Here's the drawing with two shaded views (mm, measured from the low corner). I have some questions. Round coordinates to 2 decimals unless told otherwise and drop trailing zeros. Loops run counter-clockwise (first coordinate to the right, second up) from the corner with the lowest first, then second, coordinate; pieces in that order, holes last. Notation, with made-up numbers: M -9,-32 L 49,-32 A23 cw 49,-5 Z; hole C 46,-39 d10. An arc over 180 degrees is marked long. One line per item, written item: value. Start each with the question number.
Q1. Please list where these lines run through material, in increasing order: line 1 along Y through (x, z) = (10, 31.5); line 2 along Y through (x, z) = (35, 10.5); line 3 along X through (y, z) = (11, 3.5).
Q2. Imagine slicing it at C-C (z = 8.5). Please give me the cut outline in (x, y), then the cut area to 3 significant figures.
Q3. Imagine slicing it at A-A (x = 10). Please give me the cut outline in (y, z), then the cut area to 3 significant figures.
Q4. Thinking about a two-plate mould opening in Y: for the marked faces 1, 2 and 3, which applies, released by +Y, released by -Y, zero draft, split by the parting line, or undercut?
Q5. Imagine slicing it at B-B (y = 93). Please give me the cut outline in (x, z), then the cut area to 3 significant figures.
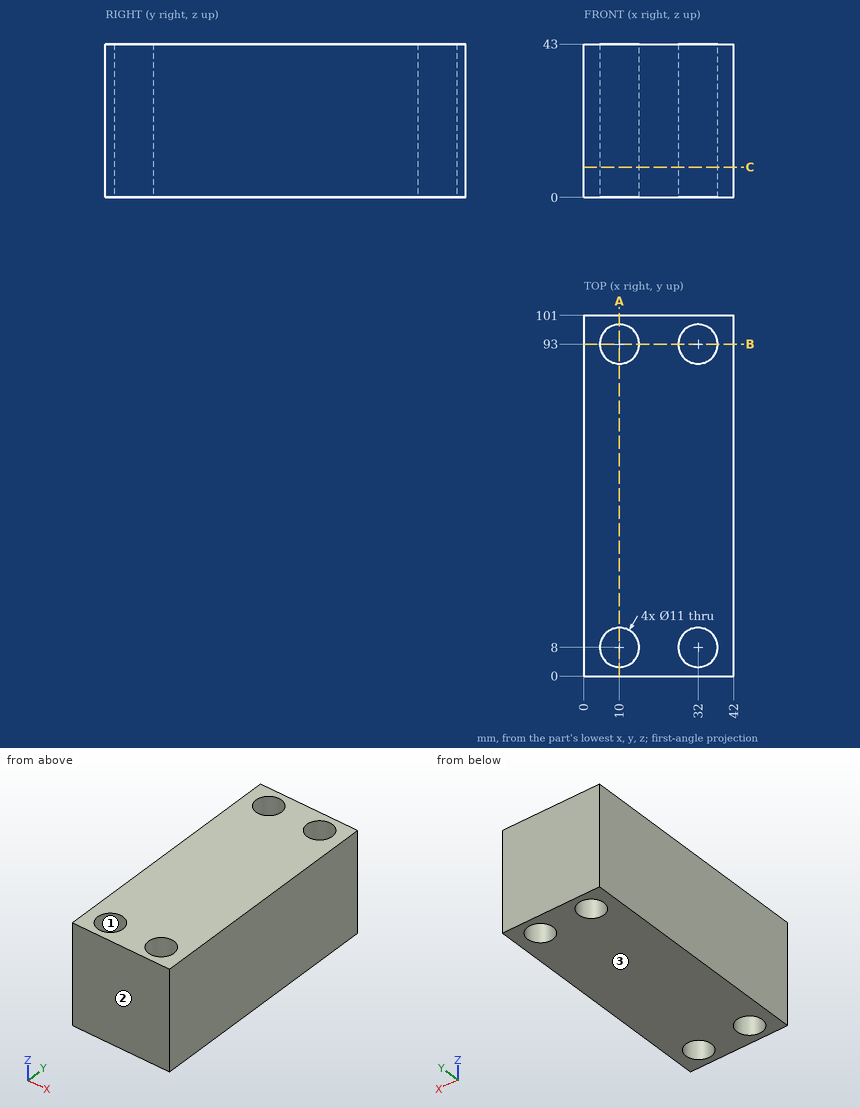
Report:
1. line 1: y = 0 to 2.5, 13.5 to 87.5, 98.5 to 101
1. line 2: y = 0 to 3.39, 12.61 to 88.39, 97.61 to 101
1. line 3: x = 0 to 5.39, 14.61 to 27.39, 36.61 to 42
2. outline: M 0,0 L 42,0 L 42,101 L 0,101 Z; hole C 10,8 d11; hole C 10,93 d11; hole C 32,8 d11; hole C 32,93 d11
2. area: 3,860 mm²
3. outline: M 0,0 L 2.5,0 L 2.5,43 L 0,43 Z; M 13.5,0 L 87.5,0 L 87.5,43 L 13.5,43 Z; M 98.5,0 L 101,0 L 101,43 L 98.5,43 Z
3. area: 3,400 mm²
4. face 1: undercut
4. face 2: released by -Y
4. face 3: zero draft
5. outline: M 0,0 L 4.5,0 L 4.5,43 L 0,43 Z; M 15.5,0 L 26.5,0 L 26.5,43 L 15.5,43 Z; M 37.5,0 L 42,0 L 42,43 L 37.5,43 Z
5. area: 860 mm²
